Here's how the part is built. I have some questions about the finished solid (model axes, mm). A direction names the side the tool comes from. Round coordinates to 2 decimals unless told otherwise and drop trailing zeros. One line per item, written item: value. Start each with the question number.
Item 1: If I drill on line 1 (Y direction, x = -11, z = 1.3) (3 decimals); line 2 (X direction, y = -46.5, z = 1.9); line 3 (X direction, y = 19, z = 0.55), over which ranges is the centre line in solid material (lowest first)?
Item 2: For P1, Ø6.5, axis at x = 17.5, y = 17.325, coming from the +Z side; P2, Ø3.5, axis at x = -5, y = 11.425, coming from the +Z side, each with a flat end and sliding along its axis, tell me the tip position at first contact or that it passes through.
Item 3: Imagine slicing it at A-A, the plane z = 4.4. Count the separate pieces of the cut face and the enclosed holes in it, then the cut area to 3 significant figures.
Item 4: For faces 4 (the face through (-11, -46.425, 3)), 5 (the face through (0, -72.325, 3)), which set-ups out of +Z, -Z, +X, -X, +Y, -Y let a thin tool reach every point of the face, with its end or its side?
Item 5: Thinking about a two-plate mould opening in X: for faces 1 (the face through (-1, -7, 5.9)), 2 (the face through (18.9, -53.82, 2.99)), 3 (the face through (-35.02, 46.8, 2.91)), which applies, released by +X, released by -X, zero draft, split by the parting line, or undercut?
```python
from build123d import *

# Parameters (mm, degrees)
SKETCH1_W           = 90
SKETCH1_H           = 154.65
SKETCH1_W_2         = 12.5
SKETCH1_H_2         = 5.9
BOSS_EXTRUDE1_DEPTH = 5.9
FILLET2_R           = 10
BOSS_EXTRUDE2_DEPTH = 5.9
CUT_EXTRUDE1_REACH  = 7.9
SKETCH5_R           = 2.05
CUT_EXTRUDE4_REACH  = 7.9
FILLET3_R           = 35


with BuildPart() as part:
    # Sketch1 → Boss-Extrude1 (new body)
    with BuildSketch(Plane.XY):
        Rectangle(SKETCH1_W, SKETCH1_H)
        with Locations((-11.25, 14.375)):
            Rectangle(SKETCH1_W_2, SKETCH1_H_2, mode=Mode.SUBTRACT)
        with Locations((11.25, 14.375)):
            Rectangle(SKETCH1_W_2, SKETCH1_H_2, mode=Mode.SUBTRACT)
        with Locations((11.25, -49.375)):
            Rectangle(SKETCH1_W_2, SKETCH1_H_2, mode=Mode.SUBTRACT)
        with Locations((-11.25, -49.375)):
            Rectangle(SKETCH1_W_2, SKETCH1_H_2, mode=Mode.SUBTRACT)
    extrude(amount=BOSS_EXTRUDE1_DEPTH)

    # Fillet2
    fillet2_edges = [part.edges().sort_by_distance(p)[0] for p in [
        (45, -77.325, 2.95),
        (-45, -77.325, 2.95),
        (-45, 77.325, 2.95),
        (45, 77.325, 2.95),
    ]]
    fillet(fillet2_edges, radius=FILLET2_R)

    # Sketch2 → Boss-Extrude2 (add)
    with BuildSketch(Plane.XY.offset(5.9)):
        Polygon((24.6, -77.325), (-24.6, -77.325), (-10, -90.939292058), (-10, -103.239292058), (-4.5, -119.325), (4.5, -119.325), (10, -103.239292058), (10, -90.939292058), align=None)
        with BuildLine():
            Line((-45, 67.325), (-45, 53.482347581))
            Line((-45, 53.482347581), (0, 77.325))
            ThreePointArc((0, 77.325), (-4.9039074, 78.609973195), (-8.547536888, 82.134661558))
            Line((-8.547536888, 82.134661558), (-15.653395136, 93.836708769))
            Line((-15.653395136, 93.836708769), (-36.605205168, 117.74389141))
            Line((-36.605205168, 117.74389141), (-44.297988367, 113.072586812))
            Line((-44.297988367, 113.072586812), (-38.587949383, 93.072586812))
            Line((-38.587949383, 93.072586812), (-31.970396029, 80.241759725))
            ThreePointArc((-31.970396029, 80.241759725), (-32.040056415, 78.284211705), (-33.747908787, 77.325))
            Line((-33.747908787, 77.325), (-35, 77.325))
            ThreePointArc((-35, 77.325), (-42.071067812, 74.396067812), (-45, 67.325))
        make_face()
        with BuildLine():
            ThreePointArc((8.547536888, 82.134661558), (4.9039074, 78.609973195), (0, 77.325))
            Line((0, 77.325), (45, 53.482347581))
            Line((45, 53.482347581), (45, 67.325))
            ThreePointArc((45, 67.325), (42.071067812, 74.396067812), (35, 77.325))
            Line((35, 77.325), (33.747908787, 77.325))
            ThreePointArc((33.747908787, 77.325), (32.040056415, 78.284211705), (31.970396029, 80.241759725))
            Line((31.970396029, 80.241759725), (38.587949383, 93.072586812))
            Line((38.587949383, 93.072586812), (44.297988367, 113.072586812))
            Line((44.297988367, 113.072586812), (36.605205168, 117.74389141))
            Line((36.605205168, 117.74389141), (15.653395136, 93.836708769))
            Line((15.653395136, 93.836708769), (8.547536888, 82.134661558))
        make_face()
    extrude(amount=-BOSS_EXTRUDE2_DEPTH)

    # Sketch5 → Cut-Extrude1 (cut, up to next)
    with BuildSketch(Plane.XY.offset(5.9), mode=Mode.PRIVATE) as cut_extrude1_sk1:
        with Locations((-17.5, 11.425)):
            Circle(SKETCH5_R)
    cut_extrude1_tool1 = extrude(cut_extrude1_sk1.sketch, amount=-CUT_EXTRUDE1_REACH, mode=Mode.PRIVATE) & part.part
    add(cut_extrude1_tool1.solids().sort_by_distance((-17.5, 11.425, 5.9))[0], mode=Mode.SUBTRACT)
    # Sketch5 → Cut-Extrude1 (cut, up to next)
    with BuildSketch(Plane.XY.offset(5.9), mode=Mode.PRIVATE) as cut_extrude1_sk2:
        with Locations((-5, 11.425)):
            Circle(SKETCH5_R)
    cut_extrude1_tool2 = extrude(cut_extrude1_sk2.sketch, amount=-CUT_EXTRUDE1_REACH, mode=Mode.PRIVATE) & part.part
    add(cut_extrude1_tool2.solids().sort_by_distance((-5, 11.425, 5.9))[0], mode=Mode.SUBTRACT)
    # Sketch5 → Cut-Extrude1 (cut, up to next)
    with BuildSketch(Plane.XY.offset(5.9), mode=Mode.PRIVATE) as cut_extrude1_sk3:
        with Locations((-5, 17.325)):
            Circle(SKETCH5_R)
    cut_extrude1_tool3 = extrude(cut_extrude1_sk3.sketch, amount=-CUT_EXTRUDE1_REACH, mode=Mode.PRIVATE) & part.part
    add(cut_extrude1_tool3.solids().sort_by_distance((-5, 17.325, 5.9))[0], mode=Mode.SUBTRACT)
    # Sketch5 → Cut-Extrude1 (cut, up to next)
    with BuildSketch(Plane.XY.offset(5.9), mode=Mode.PRIVATE) as cut_extrude1_sk4:
        with Locations((-17.5, 17.325)):
            Circle(SKETCH5_R)
    cut_extrude1_tool4 = extrude(cut_extrude1_sk4.sketch, amount=-CUT_EXTRUDE1_REACH, mode=Mode.PRIVATE) & part.part
    add(cut_extrude1_tool4.solids().sort_by_distance((-17.5, 17.325, 5.9))[0], mode=Mode.SUBTRACT)
    # Sketch5 → Cut-Extrude1 (cut, up to next)
    with BuildSketch(Plane.XY.offset(5.9), mode=Mode.PRIVATE) as cut_extrude1_sk5:
        with Locations((17.5, 11.425)):
            Circle(SKETCH5_R)
    cut_extrude1_tool5 = extrude(cut_extrude1_sk5.sketch, amount=-CUT_EXTRUDE1_REACH, mode=Mode.PRIVATE) & part.part
    add(cut_extrude1_tool5.solids().sort_by_distance((17.5, 11.425, 5.9))[0], mode=Mode.SUBTRACT)
    # Sketch5 → Cut-Extrude1 (cut, up to next)
    with BuildSketch(Plane.XY.offset(5.9), mode=Mode.PRIVATE) as cut_extrude1_sk6:
        with Locations((17.5, 17.325)):
            Circle(SKETCH5_R)
    cut_extrude1_tool6 = extrude(cut_extrude1_sk6.sketch, amount=-CUT_EXTRUDE1_REACH, mode=Mode.PRIVATE) & part.part
    add(cut_extrude1_tool6.solids().sort_by_distance((17.5, 17.325, 5.9))[0], mode=Mode.SUBTRACT)
    # Sketch5 → Cut-Extrude1 (cut, up to next)
    with BuildSketch(Plane.XY.offset(5.9), mode=Mode.PRIVATE) as cut_extrude1_sk7:
        with Locations((5, 17.325)):
            Circle(SKETCH5_R)
    cut_extrude1_tool7 = extrude(cut_extrude1_sk7.sketch, amount=-CUT_EXTRUDE1_REACH, mode=Mode.PRIVATE) & part.part
    add(cut_extrude1_tool7.solids().sort_by_distance((5, 17.325, 5.9))[0], mode=Mode.SUBTRACT)
    # Sketch5 → Cut-Extrude1 (cut, up to next)
    with BuildSketch(Plane.XY.offset(5.9), mode=Mode.PRIVATE) as cut_extrude1_sk8:
        with Locations((5, 11.425)):
            Circle(SKETCH5_R)
    cut_extrude1_tool8 = extrude(cut_extrude1_sk8.sketch, amount=-CUT_EXTRUDE1_REACH, mode=Mode.PRIVATE) & part.part
    add(cut_extrude1_tool8.solids().sort_by_distance((5, 11.425, 5.9))[0], mode=Mode.SUBTRACT)
    # Sketch5 → Cut-Extrude1 (cut, up to next)
    with BuildSketch(Plane.XY.offset(5.9), mode=Mode.PRIVATE) as cut_extrude1_sk9:
        with Locations((5, -52.325)):
            Circle(SKETCH5_R)
    cut_extrude1_tool9 = extrude(cut_extrude1_sk9.sketch, amount=-CUT_EXTRUDE1_REACH, mode=Mode.PRIVATE) & part.part
    add(cut_extrude1_tool9.solids().sort_by_distance((5, -52.325, 5.9))[0], mode=Mode.SUBTRACT)
    # Sketch5 → Cut-Extrude1 (cut, up to next)
    with BuildSketch(Plane.XY.offset(5.9), mode=Mode.PRIVATE) as cut_extrude1_sk10:
        with Locations((17.5, -52.325)):
            Circle(SKETCH5_R)
    cut_extrude1_tool10 = extrude(cut_extrude1_sk10.sketch, amount=-CUT_EXTRUDE1_REACH, mode=Mode.PRIVATE) & part.part
    add(cut_extrude1_tool10.solids().sort_by_distance((17.5, -52.325, 5.9))[0], mode=Mode.SUBTRACT)
    # Sketch5 → Cut-Extrude1 (cut, up to next)
    with BuildSketch(Plane.XY.offset(5.9), mode=Mode.PRIVATE) as cut_extrude1_sk11:
        with Locations((17.5, -46.425)):
            Circle(SKETCH5_R)
    cut_extrude1_tool11 = extrude(cut_extrude1_sk11.sketch, amount=-CUT_EXTRUDE1_REACH, mode=Mode.PRIVATE) & part.part
    add(cut_extrude1_tool11.solids().sort_by_distance((17.5, -46.425, 5.9))[0], mode=Mode.SUBTRACT)
    # Sketch5 → Cut-Extrude1 (cut, up to next)
    with BuildSketch(Plane.XY.offset(5.9), mode=Mode.PRIVATE) as cut_extrude1_sk12:
        with Locations((5, -46.425)):
            Circle(SKETCH5_R)
    cut_extrude1_tool12 = extrude(cut_extrude1_sk12.sketch, amount=-CUT_EXTRUDE1_REACH, mode=Mode.PRIVATE) & part.part
    add(cut_extrude1_tool12.solids().sort_by_distance((5, -46.425, 5.9))[0], mode=Mode.SUBTRACT)
    # Sketch5 → Cut-Extrude1 (cut, up to next)
    with BuildSketch(Plane.XY.offset(5.9), mode=Mode.PRIVATE) as cut_extrude1_sk13:
        with Locations((-5, -46.425)):
            Circle(SKETCH5_R)
    cut_extrude1_tool13 = extrude(cut_extrude1_sk13.sketch, amount=-CUT_EXTRUDE1_REACH, mode=Mode.PRIVATE) & part.part
    add(cut_extrude1_tool13.solids().sort_by_distance((-5, -46.425, 5.9))[0], mode=Mode.SUBTRACT)
    # Sketch5 → Cut-Extrude1 (cut, up to next)
    with BuildSketch(Plane.XY.offset(5.9), mode=Mode.PRIVATE) as cut_extrude1_sk14:
        with Locations((-5, -52.325)):
            Circle(SKETCH5_R)
    cut_extrude1_tool14 = extrude(cut_extrude1_sk14.sketch, amount=-CUT_EXTRUDE1_REACH, mode=Mode.PRIVATE) & part.part
    add(cut_extrude1_tool14.solids().sort_by_distance((-5, -52.325, 5.9))[0], mode=Mode.SUBTRACT)
    # Sketch5 → Cut-Extrude1 (cut, up to next)
    with BuildSketch(Plane.XY.offset(5.9), mode=Mode.PRIVATE) as cut_extrude1_sk15:
        with Locations((-17.5, -52.325)):
            Circle(SKETCH5_R)
    cut_extrude1_tool15 = extrude(cut_extrude1_sk15.sketch, amount=-CUT_EXTRUDE1_REACH, mode=Mode.PRIVATE) & part.part
    add(cut_extrude1_tool15.solids().sort_by_distance((-17.5, -52.325, 5.9))[0], mode=Mode.SUBTRACT)
    # Sketch5 → Cut-Extrude1 (cut, up to next)
    with BuildSketch(Plane.XY.offset(5.9), mode=Mode.PRIVATE) as cut_extrude1_sk16:
        with Locations((-17.5, -46.425)):
            Circle(SKETCH5_R)
    cut_extrude1_tool16 = extrude(cut_extrude1_sk16.sketch, amount=-CUT_EXTRUDE1_REACH, mode=Mode.PRIVATE) & part.part
    add(cut_extrude1_tool16.solids().sort_by_distance((-17.5, -46.425, 5.9))[0], mode=Mode.SUBTRACT)

    # Sketch7 → Cut-Extrude4 (cut, up to next)
    with BuildSketch(Plane.XY.offset(5.9), mode=Mode.PRIVATE) as cut_extrude4_sk1:
        with BuildLine():
            Line((-45, 67.325), (-45, 57.325))
            Line((-45, 57.325), (45, 57.325))
            Line((45, 57.325), (45, 67.325))
            ThreePointArc((45, 67.325), (42.071067812, 74.396067812), (35, 77.325))
            Line((35, 77.325), (33.747908787, 77.325))
            ThreePointArc((33.747908787, 77.325), (32.040056415, 78.284211705), (31.970396029, 80.241759725))
            Line((31.970396029, 80.241759725), (38.587949383, 93.072586812))
            Line((38.587949383, 93.072586812), (44.297988367, 113.072586812))
            Line((44.297988367, 113.072586812), (36.605205168, 117.74389141))
            Line((36.605205168, 117.74389141), (15.653395136, 93.836708769))
            Line((15.653395136, 93.836708769), (8.547536888, 82.134661558))
            ThreePointArc((8.547536888, 82.134661558), (0, 77.325), (-8.547536888, 82.134661558))
            Line((-8.547536888, 82.134661558), (-15.653395136, 93.836708769))
            Line((-15.653395136, 93.836708769), (-36.605205168, 117.74389141))
            Line((-36.605205168, 117.74389141), (-44.297988367, 113.072586812))
            Line((-44.297988367, 113.072586812), (-38.587949383, 93.072586812))
            Line((-38.587949383, 93.072586812), (-31.970396029, 80.241759725))
            ThreePointArc((-31.970396029, 80.241759725), (-32.040056415, 78.284211705), (-33.747908787, 77.325))
            Line((-33.747908787, 77.325), (-35, 77.325))
            ThreePointArc((-35, 77.325), (-42.071067812, 74.396067812), (-45, 67.325))
        make_face()
    cut_extrude4_tool1 = extrude(cut_extrude4_sk1.sketch, amount=-CUT_EXTRUDE4_REACH, mode=Mode.PRIVATE) & part.part
    add(cut_extrude4_tool1.solids().sort_by_distance((-34.373954, 76.241005, 5.9))[0], mode=Mode.SUBTRACT)
    # Sketch7 → Cut-Extrude4 (cut, up to next)
    with BuildSketch(Plane.XY.offset(5.9), mode=Mode.PRIVATE) as cut_extrude4_sk2:
        with BuildLine():
            Line((43.660254038, -72.325), (-43.660254038, -72.325))
            ThreePointArc((-43.660254038, -72.325), (-40, -75.985254038), (-35, -77.325))
            Line((-35, -77.325), (-24.6, -77.325))
            Line((-24.6, -77.325), (-10, -90.939292058))
            Line((-10, -90.939292058), (-10, -103.239292058))
            Line((-10, -103.239292058), (-4.5, -119.325))
            Line((-4.5, -119.325), (4.5, -119.325))
            Line((4.5, -119.325), (10, -103.239292058))
            Line((10, -103.239292058), (10, -90.939292058))
            Line((10, -90.939292058), (24.6, -77.325))
            Line((24.6, -77.325), (35, -77.325))
            ThreePointArc((35, -77.325), (40, -75.985254038), (43.660254038, -72.325))
        make_face()
    cut_extrude4_tool2 = extrude(cut_extrude4_sk2.sketch, amount=-CUT_EXTRUDE4_REACH, mode=Mode.PRIVATE) & part.part
    add(cut_extrude4_tool2.solids().sort_by_distance((0, -87.785653, 5.9))[0], mode=Mode.SUBTRACT)

    # Fillet3
    fillet3_edges = [part.edges().sort_by_distance(p)[0] for p in [
        (43.660254038, -72.325, 2.95),
        (-43.660254038, -72.325, 2.95),
        (45, 57.325, 2.95),
        (-45, 57.325, 2.95),
    ]]
    fillet(fillet3_edges, radius=FILLET3_R)


solid = part.part
```
Values follow:
1. line 1: y = -72.311 to -52.325, -46.425 to 11.425, 17.325 to 57.311
1. line 2: x = -43.78 to -19.55, -2.95 to 2.95, 19.55 to 43.78
1. line 3: x = -45 to -18.68, -16.32 to -6.18, -3.82 to 3.82, 6.18 to 16.32, 18.68 to 45
2. P1: stops at z = 5.9
2. P2: passes through
3. separate pieces: 1
3. enclosed holes: 4
3. area: 10,200 mm^2
4. face 4: +Z, -Z
4. face 5: +Z, -Z, +X, -X, -Y
5. face 1: zero draft
5. face 2: undercut
5. face 3: released by -X
